```python
from build123d import *
from OCP.BRepFilletAPI import BRepFilletAPI_MakeChamfer

# Parameters (mm, degrees)
SKETCH1_W           = 15
SKETCH1_H           = 13
SKETCH1_W_2         = 8.7
SKETCH1_H_2         = 3.4
BOSS_EXTRUDE1_DEPTH = 4
SKETCH2_W           = 8
SKETCH2_H           = 8
BOSS_EXTRUDE3_DEPTH = 4
CHAMFER1_SIZE       = 1
CHAMFER1_SIZE2      = 0.5
CHAMFER2_SIZE       = 0.5
CHAMFER2_SIZE2      = 1


with BuildPart() as part:
    # Sketch1 → Boss-Extrude1 (new body)
    with BuildSketch(Plane(origin=(0, 0, 0), x_dir=(1, 0, 0), z_dir=(0, 1, 0))):
        Rectangle(SKETCH1_W, SKETCH1_H)
        Rectangle(SKETCH1_W_2, SKETCH1_H_2, mode=Mode.SUBTRACT)
    extrude(amount=BOSS_EXTRUDE1_DEPTH)

    # Sketch2 → Boss-Extrude3 (add)
    with BuildSketch(Plane(origin=(0, 0, 0), x_dir=(1, 0, 0), z_dir=(0, 1, 0))):
        with Locations((11.5, 0)):
            Rectangle(SKETCH2_W, SKETCH2_H)
    extrude(amount=BOSS_EXTRUDE3_DEPTH)

    # Chamfer1: one chamfer whose edges measure the first distance from different faces: ONE call of the kernel's chamfer builder (chamfer() names one face for all edges)
    chamfer1_edges_1 = [part.edges().sort_by_distance(p)[0] for p in [
        (4.35, 0, 0),
    ]]
    chamfer1_side_1 = [part.faces().sort_by_distance(p)[0] for p in [
        (4.35, 2, 0),
    ]]
    chamfer1_edges_2 = [part.edges().sort_by_distance(p)[0] for p in [
        (0, 0, -1.7),
    ]]
    chamfer1_side_2 = [part.faces().sort_by_distance(p)[0] for p in [
        (0, 2, -1.7),
    ]]
    chamfer1_edges_3 = [part.edges().sort_by_distance(p)[0] for p in [
        (-4.35, 0, 0),
    ]]
    chamfer1_side_3 = [part.faces().sort_by_distance(p)[0] for p in [
        (-4.35, 2, 0),
    ]]
    chamfer1_edges_4 = [part.edges().sort_by_distance(p)[0] for p in [
        (0, 0, 1.7),
    ]]
    chamfer1_side_4 = [part.faces().sort_by_distance(p)[0] for p in [
        (0, 2, 1.7),
    ]]
    chamfer1 = BRepFilletAPI_MakeChamfer(part.part.solid().wrapped)
    for e in chamfer1_edges_1:
        chamfer1.Add(CHAMFER1_SIZE, CHAMFER1_SIZE2, e.wrapped, chamfer1_side_1[0].wrapped)  # the first distance lies on this face
    for e in chamfer1_edges_2:
        chamfer1.Add(CHAMFER1_SIZE, CHAMFER1_SIZE2, e.wrapped, chamfer1_side_2[0].wrapped)  # the first distance lies on this face
    for e in chamfer1_edges_3:
        chamfer1.Add(CHAMFER1_SIZE, CHAMFER1_SIZE2, e.wrapped, chamfer1_side_3[0].wrapped)  # the first distance lies on this face
    for e in chamfer1_edges_4:
        chamfer1.Add(CHAMFER1_SIZE, CHAMFER1_SIZE2, e.wrapped, chamfer1_side_4[0].wrapped)  # the first distance lies on this face
    add(Compound.cast(chamfer1.Shape()), mode=Mode.REPLACE)

    # Chamfer2
    chamfer2_edges = [part.edges().sort_by_distance(p)[0] for p in [
        (11.5, 0, 4),
        (11.5, 0, -4),
    ]]
    chamfer2_side = [part.faces().sort_by_distance(p)[0] for p in [
        (5.114196896, 0, 0),
    ]]
    chamfer(chamfer2_edges, length=CHAMFER2_SIZE, length2=CHAMFER2_SIZE2, reference=chamfer2_side[0])


solid = part.part
```
Geometry check sheet. Reference: the model listing, model coordinates, mm. A direction names the side the tool comes from. Coordinates: 2 decimals unless noted, no trailing zeros. Loops run counter-clockwise (first coordinate to the right, second up) from the corner with the lowest first, then second, coordinate; pieces in that order, holes last.
Item 1: Sectioned sample at D-D, the plane x = 12.5. Record the boundary of the cut face in (y, z).
Item 2: Access from +Z, -Z, +X, -X, +Y, -Y to the whole of each face (thin tool, end or side, straight path). Record for faces 1 (the face through (0, 2, 1.7)), 2 (the face through (11.444, 0.507, 3.754)), 3 (the face through (-4.6, 0.5, 0)).
Item 3: Thickness scan on line 1 (X direction, y = 1.4, z = 0.25); line 2 (Z direction, x = -1, y = 3.8); line 3 (X direction, y = 2.05, z = 4.75). Record the ranges inside material, lowest first.
Item 4: Sectioned sample at A-A, the plane x = -2. Record the boundary of the cut face in (y, z).
Item 5: Go/stop test with flat-tipped pins: pin 1 Ø0.9 at (x, y) = (12, 3) entering from -Z; pin 2 Ø0.9 at (y, z) = (2, 5.5) entering from +X; pin 3 Ø1.5 at (x, y) = (10, 2.5) entering from +Z. Record where each tip stops, or that it passes through.
Item 6: Release check for a two-part mould opening along X. For faces 4 (the face through (4.6, 0.5, 0)), 5 (the face through (7.5, 2, 5)), 6 (the face through (11.444, 0.507, -3.754)) record: released by +X, released by -X, zero draft, split by the parting line, or undercut.
Item 7: Sectioned sample at B-B, the plane z = -0.75. Record the boundary of the cut face in (x, y).
Item 8: Sectioned sample at C-C, the plane y = 2.95. Record the boundary of the cut face in (x, z).
Check result:
1. outline: (0, -3.5) - (1, -4) - (4, -4) - (4, 4) - (1, 4) - (0, 3.5) - close
2. face 1: +Y, -Y
2. face 2: +Z, +X, -Y
2. face 3: -Y
3. line 1: x = -7.5 to -4.35, 4.35 to 15.5
3. line 2: z = -6.5 to -1.7, 1.7 to 6.5
3. line 3: x = -7.5 to 7.5
4. outline: (0, -6.5) - (4, -6.5) - (4, -1.7) - (1, -1.7) - (0, -2.2) - close; (0, 2.2) - (1, 1.7) - (4, 1.7) - (4, 6.5) - (0, 6.5) - close
5. pin 1: stops at z = -4
5. pin 2: stops at x = 7.5
5. pin 3: stops at z = 4
6. face 4: undercut
6. face 5: released by +X
6. face 6: zero draft
7. outline: (-7.5, 0) - (-4.85, 0) - (-4.35, 1) - (-4.35, 4) - (-7.5, 4) - close; (4.35, 1) - (4.85, 0) - (15.5, 0) - (15.5, 4) - (4.35, 4) - close
8. outline: (-7.5, -6.5) - (7.5, -6.5) - (7.5, -4) - (15.5, -4) - (15.5, 4) - (7.5, 4) - (7.5, 6.5) - (-7.5, 6.5) - close; hole (-4.35, -1.7) - (4.35, -1.7) - (4.35, 1.7) - (-4.35, 1.7) - close
